Check sheet for the modelled part. Datum: model origin and axes. Units: mm. Coordinates: 2 decimals unless noted, no trailing zeros. Loops run counter-clockwise (first coordinate to the right, second up) from the corner with the lowest first, then second, coordinate; pieces in that order, holes last.
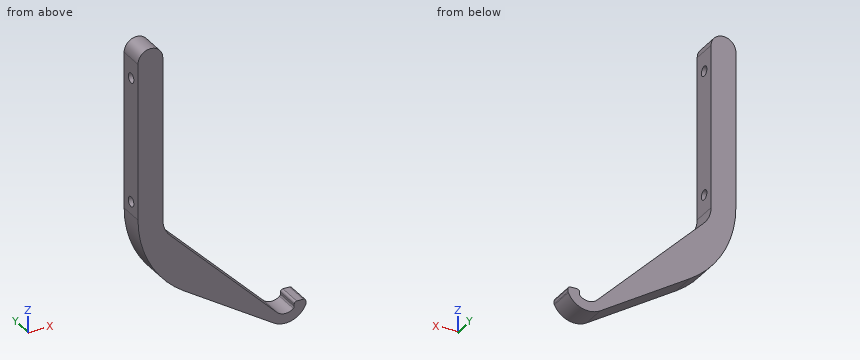
```python
from build123d import *

# Parameters (mm, degrees)
BOSS_EXTRUDE1_DEPTH = 10
SKETCH4_R           = 2
CUT_EXTRUDE3_DEPTH  = 10


with BuildPart() as part:
    # Sketch1 → Boss-Extrude1 (new body)
    with BuildSketch(Plane(origin=(0, 0, 0), x_dir=(1, 0, 0), z_dir=(0, 1, 0))):
        with BuildLine():
            Line((0, 0), (0, 53.055248535))
            ThreePointArc((0, 53.055248535), (4.930929772, 72.294799292), (18.508015666, 86.790906367))
            Line((18.508015666, 86.790906367), (54.686952948, 109.839431377))
            ThreePointArc((54.686952948, 109.839431377), (62.025319105, 110.877302623), (67.631481029, 106.029649267))
            ThreePointArc((67.631481029, 106.029649267), (67.699832136, 105.82566515), (67.722972833, 105.611782234))
            Line((67.722972833, 105.611782234), (67.722972833, 104.504374958))
            ThreePointArc((67.722972833, 104.504374958), (67.430079614, 103.797268177), (66.722972833, 103.504374958))
            Line((66.722972833, 103.504374958), (64.033008589, 103.504374958))
            ThreePointArc((64.033008589, 103.504374958), (63.325901808, 103.797268177), (63.033008589, 104.504374958))
            Line((63.033008589, 104.504374958), (63.033008589, 105.382139034))
            ThreePointArc((63.033008589, 105.382139034), (62.936856883, 105.809992118), (62.666892065, 106.155567594))
            ThreePointArc((62.666892065, 106.155567594), (59.250489983, 107.282320922), (55.961940777, 105.823958698))
            Line((55.961940777, 105.823958698), (12.928932188, 62.790950109))
            ThreePointArc((12.928932188, 62.790950109), (10.761204675, 59.546716621), (10, 55.719882297))
            Line((10, 55.719882297), (10, -0.137982079))
            Line((10, -0.137982079), (10, -10))
            ThreePointArc((10, -10), (5, -15), (0, -10))
            Line((0, -10), (0, 0))
        make_face()
    extrude(amount=BOSS_EXTRUDE1_DEPTH)

    # Sketch4 → Cut-Extrude3 (cut)
    with BuildSketch(Plane.ZY):
        with Locations((-48.055248535, 5)):
            Circle(SKETCH4_R)
        with Locations((2, 5)):
            Circle(SKETCH4_R)
    extrude(amount=-CUT_EXTRUDE3_DEPTH, mode=Mode.SUBTRACT)


solid = part.part
```
1) Section check C-C on x = 5. Enter the section's corners in (y, z).
Answer sheet:
outline: (0, -72.42) - (10, -72.42) - (10, 15) - (0, 15) - close; hole circle Ø4 at (5, -48.06); hole circle Ø4 at (5, 2)
2) Section check A-A on y = 5. Enter the section's corners in (x, z), plus the area to 3 significant figures.
Answer sheet:
outline: (0, -53.06) arc R40 ccw to (18.51, -86.79) - (54.69, -109.84) arc R8.95 ccw to (67.63, -106.03) arc R1 ccw to (67.72, -105.61) - (67.72, -104.5) arc R1 ccw to (66.72, -103.5) - (64.03, -103.5) arc R1 ccw to (63.03, -104.5) - (63.03, -105.38) arc R1 cw to (62.67, -106.16) arc R5 cw to (55.96, -105.82) - (12.93, -62.79) arc R10 cw to (10, -55.72) - (10, -50.06) - (0, -50.06) - close; (0, -46.06) - (10, -46.06) - (10, 0) - (0, 0) - close; (0, 4) - (10, 4) - (10, 10) arc R5 ccw to (0, 10) - close
area: 1,430 mm2
3) Scan lines: line 1 (Y direction, x = 2, z = 2); line 2 (X direction, y = 5, z = -36); line 3 (X direction, y = 8.75, z = -79.5). Record each from-to range of solid material in increasing order.
Answer sheet:
line 1: y = 0 to 3, 7 to 10
line 2: x = 0 to 10
line 3: x = 9.99 to 29.64
4) Section check B-B on z = 2. Enter the section's corners in (x, y), plus the area to 3 significant figures.
Answer sheet:
outline: (0, 0) - (10, 0) - (10, 3) - (0, 3) - close; (0, 7) - (10, 7) - (10, 10) - (0, 10) - close
area: 60.0 mm2
5) Section check D-D on x = 22.5. Enter the section's corners in (y, z).
Answer sheet:
outline: (0, -89.33) - (10, -89.33) - (10, -72.36) - (0, -72.36) - close
6) Depth check by flat-ended pin: pin 1 (3 mm diameter, centred on y = 4.5, z = -25.5, fed in from +X); pin 2 (4 mm diameter, centred on x = 53, y = 5.5, fed in from +Z); pin 3 (2.5 mm diameter, centred on y = 5, z = 2, fed in from +X); pin 4 (4 mm diameter, centred on x = 33, z = -91.5, fed in from -Y). Enter the tip coordinate at first touch or a pass-through.
Answer sheet:
pin 1: stops at x = 10
pin 2: stops at z = -100.86
pin 3: passes through
pin 4: stops at y = 0
